Answer from the drawing. Dimensions are ordinates in mm from the lowest x, y and z of the part. A direction names the side the tool comes from. Give positions to 0.01 mm unless a question says otherwise; leave off trailing zeros. Order: outer loops, then holes, each group sorted by start corner. A loop starts at its lowest first (then second) coordinate and runs counter-clockwise, first axis right, second up. Notation, with made-up numbers: (-36, -28) - (-16, -28) arc R19 cw to (-16, 6) - close; hole circle Ø6 at (72, -26.75). An arc over 180 degrees is marked (long way). Use a Markdown table: item, result. Add a question column.
1) The mould has two halves that part along X. Classify the marked faces 4, 5 and 6: released by +X, released by -X, zero draft, split by the parting line, or undercut.
2) Find section A-A, the plane x = 22.5. Determine the outline of the cut face in (y, z), plus the area to 3 significant figures.
3) Find section D-D, the plane y = 3. Determine the outline of the cut face in (x, z), plus the area to 3 significant figures.
4) Flat-ended cylindrical pins translate along their axes: pin 1 (1.1 mm diameter, centred on y = 9, z = 17, fed in from -X); pin 2 (10 mm diameter, centred on x = 28, z = 32, fed in from -Y); pin 3 (4 mm diameter, centred on y = 21, z = 10.5, fed in from -X); pin 4 (6 mm diameter, centred on x = 30, y = 21, fed in from +Z). Find the tip coordinate at first contact, or state that the pin passes through.
5) Find section C-C, the plane z = 8. Determine the outline of the cut face in (x, y).
6) For the marked faces 1, 2 and 3, determine the directions among +Z, -Z, +X, -X, +Y, -Y from which every point of the face is accessible in a straight line to the end or side of a thin tool.
7) Find section B-B, the plane y = 22.5. Determine the outline of the cut face in (x, z), plus the area to 3 significant figures.
8) Straight lines are drawn through the part: line 1 (Y direction, x = 22.5, z = 26); line 2 (Y direction, x = 22.5, z = 36.5); line 3 (X direction, y = 22.5, z = 23). For each, find the intervals that lie inside material, in ascending order.
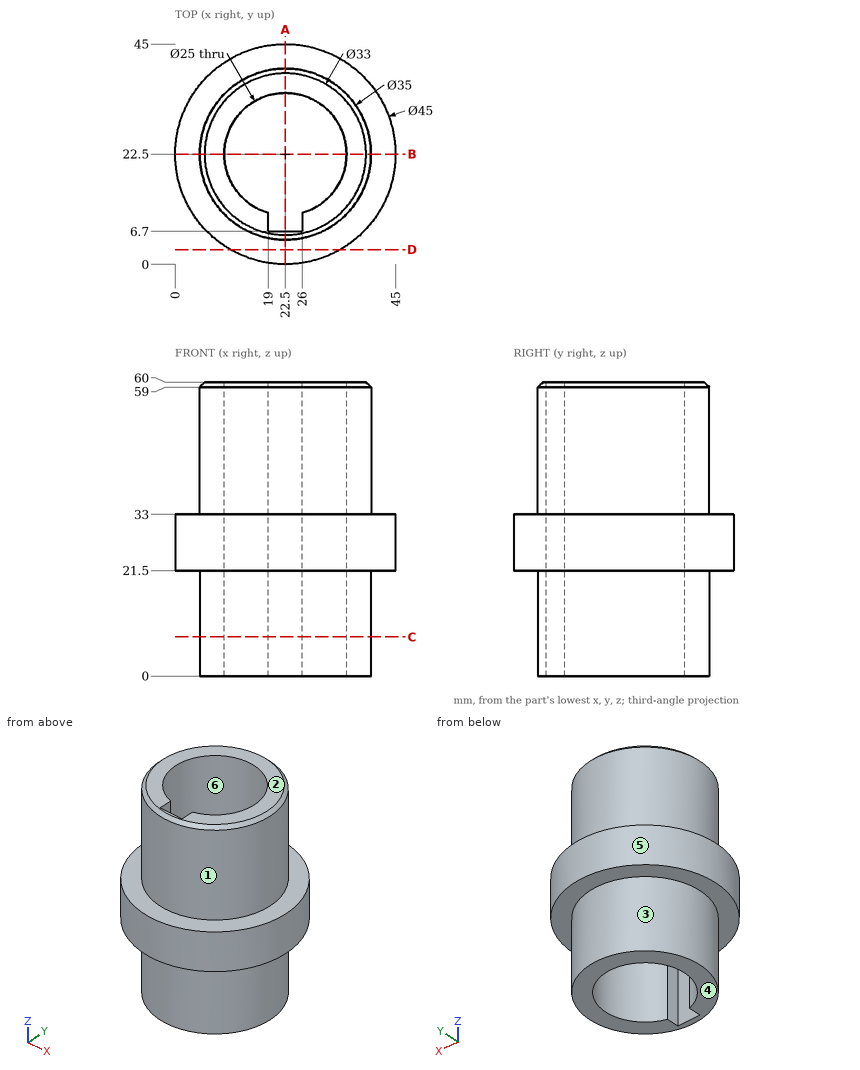
The answers:
| question | item | result |
|---|---|---|
| 1 | face 4 | zero draft |
| 1 | face 5 | split by the parting line |
| 1 | face 6 | undercut |
| 2 | outline | (0, 21.5) - (5, 21.5) - (5, 0) - (6.7, 0) - (6.7, 60) - (6, 60) - (5, 59) - (5, 33) - (0, 33) - close; (35, 0) - (40, 0) - (40, 21.5) - (45, 21.5) - (45, 33) - (40, 33) - (40, 59) - (39, 60) - (35, 60) - close |
| 2 | area | 516 mm2 |
| 3 | outline | (11.28, 21.5) - (33.72, 21.5) - (33.72, 33) - (11.28, 33) - close |
| 3 | area | 258 mm2 |
| 4 | pin 1 | x = 10.73 |
| 4 | pin 2 | y = 0.01 |
| 4 | pin 3 | x = 5 |
| 4 | pin 4 | through |
| 5 | outline | circle Ø35 at (22.5, 22.5); hole (19, 6.7) - (26, 6.7) - (26, 10.5) arc R12.5 ccw (long way) to (19, 10.5) - close |
| 6 | face 1 | +Z |
| 6 | face 2 | +Z, +X, -X, +Y, -Y |
| 6 | face 3 | -Z |
| 7 | outline | (0, 21.5) - (5, 21.5) - (5, 0) - (10, 0) - (10, 60) - (6, 60) - (5, 59) - (5, 33) - (0, 33) - close; (35, 0) - (40, 0) - (40, 21.5) - (45, 21.5) - (45, 33) - (40, 33) - (40, 59) - (39, 60) - (35, 60) - close |
| 7 | area | 714 mm2 |
| 8 | line 1 | 0 to 6.7, 35 to 45 |
| 8 | line 2 | 5 to 6.7, 35 to 40 |
| 8 | line 3 | 0 to 10, 35 to 45 |
